Build history of the part. All positions in model axes, mm. Coordinates: 2 decimals unless noted, no trailing zeros. Write each loop counter-clockwise with the first axis right and the second up, starting at its lowest first coordinate (ties: lowest second). Pieces come first, ordered by that corner, then holes.
```python
from build123d import *

# Parameters (mm, degrees)
BOSS_EXTRUDE1_DEPTH   = 12.7
F_6_CLEARANCE_HOLE2_D = 3.7973
F_6_CLEARANCE_HOLE1_D = 3.7973


with BuildPart() as part:
    # Sketch1 → Boss-Extrude1 (new body)
    with BuildSketch(Plane(origin=(0, 0, 0), x_dir=(1, 0, 0), z_dir=(0, 1, 0))):
        Polygon((0, -5.255172414), (0, 20.144827586), (25.4, 20.144827586), (25.4, 18.557327586), (1.5875, 18.557327586), (1.5875, -5.255172414), align=None)
    extrude(amount=BOSS_EXTRUDE1_DEPTH)

    # #6 Clearance Hole2 (through all)
    with Locations(Plane(origin=(1.5875, 0, 0), x_dir=(0, 0, -1), z_dir=(1, 0, 0))):
        with Locations((7.444827586, 6.35)):
            Hole(F_6_CLEARANCE_HOLE2_D / 2)

    # #6 Clearance Hole1 (through all)
    with Locations(Plane.XY.offset(-18.557327586)):
        with Locations((12.7, 6.35)):
            Hole(F_6_CLEARANCE_HOLE1_D / 2)


solid = part.part
```
1. Saw through at B-B on y = 6.35. List the corners of the cut face in (x, z), plus the area to 3 significant figures.
Computed values:
outline: (0, -20.14) - (10.8, -20.14) - (10.8, -18.56) - (1.59, -18.56) - (1.59, -9.34) - (0, -9.34) - close; (0, -5.55) - (1.59, -5.55) - (1.59, 5.26) - (0, 5.26) - close; (14.6, -20.14) - (25.4, -20.14) - (25.4, -18.56) - (14.6, -18.56) - close
area: 66.1 mm2
2. Flat gauge pins, fed straight in: pin 1 (2 mm diameter, centred on x = 20.5, y = 11, fed in from +Z); pin 2 (4 mm diameter, centred on y = 8.5, z = -8, fed in from +X). Where does each tip first touch, or does it go through?
Computed values:
pin 1: stops at z = -18.56
pin 2: stops at x = 1.59
3. Saw through at C-C on y = 1.75. List the corners of the cut face in (x, z), plus the area to 3 significant figures.
Computed values:
outline: (0, -20.14) - (25.4, -20.14) - (25.4, -18.56) - (1.59, -18.56) - (1.59, 5.26) - (0, 5.26) - close
area: 78.1 mm2
4. Saw through at A-A on x = 12.7. List the corners of the cut face in (y, z), plus the area to 3 significant figures.
Computed values:
outline: (0, -20.14) - (4.45, -20.14) - (4.45, -18.56) - (0, -18.56) - close; (8.25, -20.14) - (12.7, -20.14) - (12.7, -18.56) - (8.25, -18.56) - close
area: 14.1 mm2
5. Saw through at D-D on z = -4. List the corners of the cut face in (x, y), plus the area to 3 significant figures.
Computed values:
outline: (0, 0) - (1.59, 0) - (1.59, 12.7) - (0, 12.7) - close
area: 20.2 mm2
6. Mould opens along Z. For faces 1 (the face through (15, 6, -20.145)), 2 (the face through (16, 6, -18.557)), 3 (the face through (0.8, 5.6, -5.7)), 4 (the face through (1.588, 6, -4)) say: +Z half, -Z half, draft (parallel to the pull), parting line (faces both ways), or undercut.
Computed values:
face 1: -Z half
face 2: +Z half
face 3: undercut
face 4: draft
7. Probe line 1 along Y through (x, z) = (12.7, -19.4); line 2 along X through (y, z) = (10, -17); line 3 along Z through (x, y) = (17.5, 7). List the from-to ranges inside material, lowest first.
Computed values:
line 1: y = 0 to 4.45, 8.25 to 12.7
line 2: x = 0 to 1.59
line 3: z = -20.14 to -18.56
